The listing builds one solid part. Answer for the finished solid, in the listing's coordinates (mm). Face numbers are marked on the shaded views. Give positions to 0.01 mm unless a question says otherwise; leave off trailing zeros. Order: outer loops, then holes, each group sorted by start corner. A loop starts at its lowest first (then second) coordinate and runs counter-clockwise, first axis right, second up. Notation, with made-up numbers: (12, 74) -> (64, 74) arc R12 cw to (64, 97) -> close; hole circle Ø4 at (37.5, 13). An arc over 180 degrees is marked (long way). Answer as a JSON object with one key per item and string values. Group by question number.
```python
from build123d import *

# Parameters (mm, degrees)
SKETCH2_R           = 2
BOSS_EXTRUDE1_DEPTH = 10
CUT_EXTRUDE1_DEPTH  = 1.5


with BuildPart() as part:
    # Sketch1 → Revolve1 (revolve)
    with BuildSketch(Plane(origin=(0, 0, 0), x_dir=(0, 0, -1), z_dir=(1, 0, 0))):
        with BuildLine():
            Line((0, 0), (0, 2.2))
            Line((0, 2.2), (-1.25, 2.2))
            ThreePointArc((-1.25, 2.2), (-2.80380946, 1.466174172), (-3.7, 0))
            Line((-3.7, 0), (0, 0))
        make_face()
    revolve(axis=Axis((0, 4.725289413, 0), (0, -1, 0)))

    # Sketch2 → Boss-Extrude1 (add)
    with BuildSketch(Plane.XZ):
        Circle(SKETCH2_R)
    extrude(amount=BOSS_EXTRUDE1_DEPTH)

    # Sketch3 → Cut-Extrude1 (cut)
    with BuildSketch(Plane(origin=(0, 2.2, 0), x_dir=(1, 0, 0), z_dir=(0, 1, 0))):
        Polygon((0, 1.25), (-1.082531755, 0.625), (-1.082531755, -0.625), (0, -1.25), (1.082531755, -0.625), (1.082531755, 0.625), align=None)
    extrude(amount=-CUT_EXTRUDE1_DEPTH, mode=Mode.SUBTRACT)


solid = part.part
```
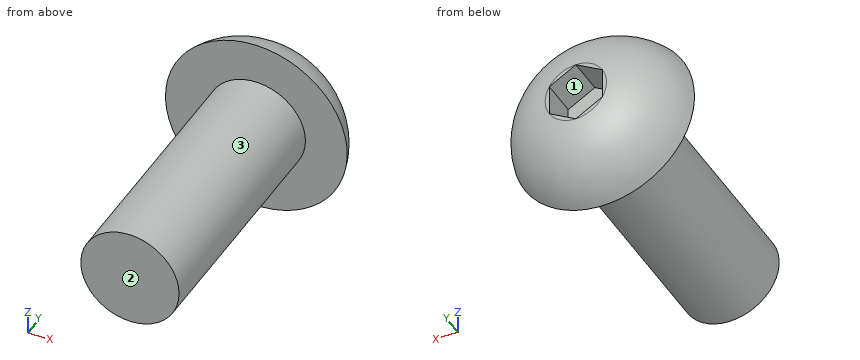
(1) Flat-ended cylindrical pins translate along their axes: pin 1 Ø1 at (x, y) = (-1, -3.5) entering from +Z; pin 2 Ø0.6 at (y, z) = (1.5, -0.5) entering from -X; pin 3 Ø2 at (x, y) = (-0.5, -7) entering from +Z. Find the tip coordinate at first contact, or state that the pin passes through.
(2) A cutting plane is placed at A-A (y = -1). Determine the outline of the cut face in (x, z).
(3) For a pull along Z with two mould halves and no side action, classify the marked faces 1, 2 and 3 as +Z half, -Z half, draft (parallel to the pull), parting line (faces both ways), or undercut.
(4) Find the intervals of material crossed by line 1 along Y through (x, z) = (-1.75, -0.75); line 2 along X through (y, z) = (-9.25, 1.5); line 3 along Y through (x, z) = (-1, -1.25), in increasing order. Write a range as [from, to].
Check sheet entries:
{
 "1": {"pin 1": "stops at z = 1.94", "pin 2": "stops at x = -3.03", "pin 3": "stops at z = 2"},
 "2": {"outline": "circle Ø4 at (0, 0)"},
 "3": {"face 1": "undercut", "face 2": "draft", "face 3": "parting line"},
 "4": {"line 1": "y = [-10, 2.02]", "line 2": "x = [-1.32, 1.32]", "line 3": "y = [-10, 2.13]"}
}
